Could you check a few things on this model? Use its own coordinates, in mm. A direction names the side the tool comes from. Round coordinates to 2 decimals unless told otherwise and drop trailing zeros. Write each loop counter-clockwise with the first axis right and the second up, starting at its lowest first coordinate (ties: lowest second). Pieces come first, ordered by that corner, then holes.
```python
from build123d import *

# Parameters (mm, degrees)
BOSS_EXTRUDE5_DEPTH = 10
BOSS_EXTRUDE6_DEPTH = 14.5
BOSS_EXTRUDE7_REACH = 63.425
SKETCH28_W          = 11
SKETCH28_H          = 29
SKETCH37_W          = 23.2
SKETCH37_H          = 14.666666667
CUT_EXTRUDE10_DEPTH = 6
SKETCH38_W          = 23.2
SKETCH38_H          = 5
CUT_EXTRUDE11_DEPTH = 6
SKETCH39_R          = 1.05
CUT_EXTRUDE12_DEPTH = 81.736980805
SKETCH40_R          = 2
CUT_EXTRUDE13_DEPTH = 1.4
SKETCH41_R          = 2
CUT_EXTRUDE14_DEPTH = 1.4
SKETCH42_W          = 17
SKETCH42_H          = 40
CUT_EXTRUDE15_DEPTH = 77.175521458
FILLET2_R           = 2
CUT_EXTRUDE16_DEPTH = 80.232001549
BOSS_EXTRUDE8_DEPTH = 10
FILLET3_R           = 10
FILLET4_R           = 5.45


with BuildPart() as part:
    # Sketch25 → Boss-Extrude5 (new, symmetric)
    with BuildSketch(Plane.XY):
        with BuildLine():
            Line((0, 15.875), (6.35, 15.875))
            ThreePointArc((6.35, 15.875), (9.840958299, 0), (6.35, -15.875))
            Line((6.35, -15.875), (0, -15.875))
            ThreePointArc((0, -15.875), (4.187196601, 0), (0, 15.875))
        make_face()
    extrude(amount=BOSS_EXTRUDE5_DEPTH, both=True)


with BuildPart() as body_2:
    # Sketch27 → Boss-Extrude6 (new, symmetric)
    with BuildSketch(Plane.XY):
        Polygon((0, -30.541666667), (11, -30.541666667), (11, -74.541666667), (0, -74.541666667), (0, -69.541666667), (6, -69.541666667), (6, -35.541666667), (0, -35.541666667), align=None)
    extrude(amount=BOSS_EXTRUDE6_DEPTH, both=True)

    # Sketch28 → Boss-Extrude7 (add, up to next)
    with BuildSketch(Plane.XZ.offset(15.875), mode=Mode.PRIVATE) as boss_extrude7_sk1:
        with Locations((5.5, 0)):
            Rectangle(SKETCH28_W, SKETCH28_H)
    boss_extrude7_tool1 = extrude(boss_extrude7_sk1.sketch, amount=BOSS_EXTRUDE7_REACH, mode=Mode.PRIVATE) - body_2.part

    add(part.part)  # Boss-Extrude7 merges part
    add(boss_extrude7_tool1.solids().sort_by_distance((5.5, -15.875, 0))[0])

    # Sketch37 → Cut-Extrude10 (cut)
    with BuildSketch(Plane.ZY):
        with Locations((0, -28.208333334)):
            Rectangle(SKETCH37_W, SKETCH37_H)
    extrude(amount=-CUT_EXTRUDE10_DEPTH, mode=Mode.SUBTRACT)

    # Sketch38 → Cut-Extrude11 (cut)
    with BuildSketch(Plane.ZY):
        with Locations((0, -72.041666667)):
            Rectangle(SKETCH38_W, SKETCH38_H)
    extrude(amount=-CUT_EXTRUDE11_DEPTH, mode=Mode.SUBTRACT)

    # Sketch39 → Cut-Extrude12 (cut, through all)
    with BuildSketch(Plane(origin=(0, 0, -14.5), x_dir=(-1, 0, 0), z_dir=(0, 0, -1))):
        with Locations((-2.5, -33.041666667)):
            Circle(SKETCH39_R)
        with Locations((-2.5, -72.041666667)):
            Circle(SKETCH39_R)
    extrude(amount=-CUT_EXTRUDE12_DEPTH, mode=Mode.SUBTRACT)

    # Sketch40 → Cut-Extrude13 (cut)
    with BuildSketch(Plane(origin=(0, 0, -14.5), x_dir=(-1, 0, 0), z_dir=(0, 0, -1))):
        with Locations((-2.5, -33.041666667)):
            Circle(SKETCH40_R)
        with Locations((-2.5, -72.041666667)):
            Circle(SKETCH40_R)
    extrude(amount=-CUT_EXTRUDE13_DEPTH, mode=Mode.SUBTRACT)

    # Sketch41 → Cut-Extrude14 (cut)
    with BuildSketch(Plane.XY.offset(14.5)):
        with Locations(Location((2.5, -33.041666667, 0), (0, 0, 180))):
            Circle(SKETCH41_R)
        with Locations(Location((2.5, -72.041666667, 0), (0, 0, 180))):
            Circle(SKETCH41_R)
    extrude(amount=-CUT_EXTRUDE14_DEPTH, mode=Mode.SUBTRACT)

    # Sketch42 → Cut-Extrude15 (cut, through all)
    with BuildSketch(Plane.ZY.offset(-6)):
        with Locations((0, -49.541666667)):
            Rectangle(SKETCH42_W, SKETCH42_H)
    extrude(amount=-CUT_EXTRUDE15_DEPTH, mode=Mode.SUBTRACT)

    # Fillet2
    fillet2_edges = [body_2.edges().sort_by_distance(p)[0] for p in [
        (8.5, -69.541666667, -8.5),
        (8.5, -29.541666667, -8.5),
        (8.5, -29.541666667, 8.5),
        (8.5, -69.541666667, 8.5),
        (0, -35.541666667, 13.05),
        (0, -69.541666667, 13.05),
        (0, -74.541666667, 13.05),
        (11, -74.541666667, 0),
        (0, -35.541666667, -13.05),
        (0, -74.541666667, -13.05),
        (0, -69.541666667, -13.05),
    ]]
    fillet(fillet2_edges, radius=FILLET2_R)

    # Sketch44 → Cut-Extrude16 (cut, through all)
    with BuildSketch(Plane.XY.offset(10)):
        with BuildLine():
            Line((6.35, -15.875), (0, -15.875))
            ThreePointArc((0, -15.875), (4.187196601, 0), (0, 15.875))
            Line((0, 15.875), (6.35, 15.875))
            ThreePointArc((6.35, 15.875), (9.840958299, 0), (6.35, -15.875))
        make_face()
    extrude(amount=-CUT_EXTRUDE16_DEPTH, mode=Mode.SUBTRACT)

    # Sketch43 → Boss-Extrude8 (add, symmetric)
    with BuildSketch(Plane.XY):
        with BuildLine():
            Line((-3.25, 15.875), (3.1, 15.875))
            ThreePointArc((3.1, 15.875), (6.232422098, 0), (3.1, -15.875))
            Line((3.1, -15.875), (-3.25, -15.875))
            ThreePointArc((-3.25, -15.875), (0.439252949, 0), (-3.25, 15.875))
        make_face()
    extrude(amount=BOSS_EXTRUDE8_DEPTH, both=True)

    # Fillet3
    # the kernel refuses this fillet: 10 mm, written as the material it takes off along each edge
    with BuildSketch(Plane(origin=(11, -15.875, 39.5), x_dir=(-1, 0, 0), z_dir=(0, 0, -1))) as fillet3_piece_1_section:
        with BuildLine():
            CenterArc((FILLET3_R, -FILLET3_R), FILLET3_R, 90, 90)
            Line((0, -FILLET3_R), (0, 0))
            Line((0, 0), (FILLET3_R, 0))
        make_face()
    fillet3_piece_1 = extrude(amount=79, mode=Mode.PRIVATE)
    fillet3_piece_1 = split(fillet3_piece_1, bisect_by=Plane(origin=(2.190951885, -15.815672455, 10), z_dir=(0, 0, 1)), keep=Keep.TOP, mode=Mode.PRIVATE)
    fillet3_piece_1 = fillet3_piece_1 & Plane(origin=(-35.560747051, 0, 24.75), x_dir=(0.925049424055658, 0.3798467625955178, 0), z_dir=(0, 0, 1)) * Cylinder(41.793169149, 198, mode=Mode.PRIVATE)
    add(fillet3_piece_1, mode=Mode.SUBTRACT)
    with BuildSketch(Plane(origin=(11, -15.875, 39.5), x_dir=(-1, 0, 0), z_dir=(0, 0, -1))) as fillet3_piece_2_section:
        with BuildLine():
            CenterArc((FILLET3_R, -FILLET3_R), FILLET3_R, 90, 90)
            Line((0, -FILLET3_R), (0, 0))
            Line((0, 0), (FILLET3_R, 0))
        make_face()
    fillet3_piece_2 = extrude(amount=79, mode=Mode.PRIVATE)
    fillet3_piece_2 = split(fillet3_piece_2, bisect_by=Plane(origin=(8.886802667, -18.192463431, 10), z_dir=(0, 0, 1)), keep=Keep.TOP, mode=Mode.PRIVATE)
    fillet3_piece_2 = fillet3_piece_2 - Plane(origin=(-35.560747051, 0, 24.75), x_dir=(0.925049424055658, 0.3798467625955178, 0), z_dir=(0, 0, 1)) * Cylinder(41.793169149, 198, mode=Mode.PRIVATE)
    add(fillet3_piece_2, mode=Mode.SUBTRACT)
    with BuildSketch(Plane(origin=(11, -15.875, 39.5), x_dir=(-1, 0, 0), z_dir=(0, 0, -1))) as fillet3_piece_3_section:
        with BuildLine():
            CenterArc((FILLET3_R, -FILLET3_R), FILLET3_R, 90, 90)
            Line((0, -FILLET3_R), (0, 0))
            Line((0, 0), (FILLET3_R, 0))
        make_face()
    fillet3_piece_3 = extrude(amount=79, mode=Mode.PRIVATE)
    fillet3_piece_3 = split(fillet3_piece_3, bisect_by=Plane(origin=(8.886802667, -18.192463431, 10), z_dir=(0, 0, -1)), keep=Keep.TOP, mode=Mode.PRIVATE)
    fillet3_piece_3 = fillet3_piece_3 - Plane(origin=(-35.560747051, 0, 0), x_dir=(0.925049424055658, 0.3798467625955178, 0), z_dir=(0, 0, 1)) * Cylinder(41.793169149, 198, mode=Mode.PRIVATE)
    fillet3_piece_3 = split(fillet3_piece_3, bisect_by=Plane(origin=(8.886802667, -18.192463431, -10), z_dir=(0, 0, 1)), keep=Keep.TOP, mode=Mode.PRIVATE)
    add(fillet3_piece_3, mode=Mode.SUBTRACT)
    with BuildSketch(Plane(origin=(11, -15.875, 39.5), x_dir=(-1, 0, 0), z_dir=(0, 0, -1))) as fillet3_piece_4_section:
        with BuildLine():
            CenterArc((FILLET3_R, -FILLET3_R), FILLET3_R, 90, 90)
            Line((0, -FILLET3_R), (0, 0))
            Line((0, 0), (FILLET3_R, 0))
        make_face()
    fillet3_piece_4 = extrude(amount=79, mode=Mode.PRIVATE)
    fillet3_piece_4 = fillet3_piece_4 & Plane(origin=(-35.560747051, 0, -24.75), x_dir=(0.925049424055658, 0.3798467625955178, 0), z_dir=(0, 0, 1)) * Cylinder(41.793169149, 198, mode=Mode.PRIVATE)
    fillet3_piece_4 = split(fillet3_piece_4, bisect_by=Plane(origin=(2.190951885, -15.815672455, -10), z_dir=(0, 0, -1)), keep=Keep.TOP, mode=Mode.PRIVATE)
    add(fillet3_piece_4, mode=Mode.SUBTRACT)
    with BuildSketch(Plane(origin=(11, -15.875, 39.5), x_dir=(-1, 0, 0), z_dir=(0, 0, -1))) as fillet3_piece_5_section:
        with BuildLine():
            CenterArc((FILLET3_R, -FILLET3_R), FILLET3_R, 90, 90)
            Line((0, -FILLET3_R), (0, 0))
            Line((0, 0), (FILLET3_R, 0))
        make_face()
    fillet3_piece_5 = extrude(amount=79, mode=Mode.PRIVATE)
    fillet3_piece_5 = fillet3_piece_5 - Plane(origin=(-35.560747051, 0, -24.75), x_dir=(0.925049424055658, 0.3798467625955178, 0), z_dir=(0, 0, 1)) * Cylinder(41.793169149, 198, mode=Mode.PRIVATE)
    fillet3_piece_5 = split(fillet3_piece_5, bisect_by=Plane(origin=(8.886802667, -18.192463431, -10), z_dir=(0, 0, -1)), keep=Keep.TOP, mode=Mode.PRIVATE)
    add(fillet3_piece_5, mode=Mode.SUBTRACT)

    # Fillet4
    # the kernel refuses this fillet: 5.45 mm, written as the material it adds along each edge
    with BuildSketch(Plane(origin=(0, -15.875, 10), x_dir=(-1, 0, 0), z_dir=(0, 0, -1))) as fillet4_piece_1:
        with BuildLine():
            CenterArc((5.45, -4.986231042), FILLET4_R, 113.807792078, 66.192207922)
            Line((0, -4.986231042), (0, 0))
            Line((0, 0), (3.25, 0))
        make_face()
    extrude(amount=20)
    with BuildSketch(Plane(origin=(3.015126937, -16.080140969, -10), x_dir=(0.33239794280209367, 0.9431392302417156, 0), z_dir=(0, 0, 1))) as fillet4_piece_2:
        with BuildLine():
            CenterArc((4.992113304, -5.441426809), FILLET4_R, 93.214160673, 71.449916977)
            ThreePointArc((-0.263821953, -4.000023125), (0.07058047, -2.013366907), (0, 0))
            ThreePointArc((0, 0), (2.343270621, -0.065743272), (4.686541241, 0))
        make_face()
    extrude(amount=20)


solid = body_2.part
```
Q1. If I drill on L1, parallel to Z at x = 8, y = -39.5; L2, parallel to Y at x = 2.5, z = 12.3; L3, parallel to Z at x = 5.5, y = -34, over which ranges is the centre line in solid material (lowest first)?
Q2. I'm going to push flat-ended pins straight in: pin 1 Ø2 at (x, y) = (2.5, -34) entering from -Z; pin 2 Ø1.5 at (x, z) = (4, -12.5) entering from +Y; pin 3 Ø1.3 at (x, y) = (2.5, -33.04) entering from -Z; pin 4 Ø5 at (y, z) = (-12.5, 2.5) entering from -X. Where does each tip first touch, or does it pass through?
Q3. On a 3-axis mill with a long thin cutter (end or side, diameter ignored), from which of +Z, -Z, +X, -X, +Y, -Y can I reach the whole of each face in a straight line? I mean faces 4 (the cylindrical face through (2.76, -31.06, -13.81)), 5 (the flat face through (8, -50, -8.5)), 6 (the flat face through (3, -28, -11.6)), 7 (the cylindrical face through (0.57, -70.143, 13.03)), 8 (the flat face through (1.6, -71.2, 13.1)). Say none if no direction works.
Q4. Imagine slicing it at B-B, the plane z = 1. Write out the boundary of the cut face in (x, y) (3 decimals), then the cut area to 3 significant figures.
Q5. We'd pull the mould along Z, two halves only. Please class faces 1 (the flat face through (4, -69.542, 13)), 2 (the flat face through (7, -45, 14.5)), 3 (the cylindrical face through (8.535, -30.143, 7.93)): pulls with the +Z half, pulls with the -Z half, needs draft (parallel to the pull), parting line crosses it, or undercut.
Q6. Imagine slicing it at A-A, the plane y = -51.5. Write out the boundary of the cut face in (x, z).
Q7. Imagine slicing it at D-D, the plane y = -14. Write out the boundary of the cut face in (x, z).
Q8. Imagine slicing it at C-C, the plane y = 2. Write out the boundary of the cut face in (x, z), then the cut area to 3 significant figures.
Results found:
1. L1: z = -14.5 to -8.5, 8.5 to 14.5
1. L2: y = -74.54 to -73.09, -70.99 to -69.54, -35.54 to -34.09, -31.99 to -15.99
1. L3: z = -14.5 to -11.6, 11.6 to 14.5
2. pin 1: stops at z = -13.1
2. pin 2: stops at y = -16.13
2. pin 3: passes through
2. pin 4: stops at x = -2.83
3. face 4: -Z
3. face 5: +X, -X
3. face 6: -X, -Y
3. face 7: +Z, -Z, -X
3. face 8: +Z
4. outline: (-3.25, -15.875) arc R5.45 cw to (0, -20.861) - (0, -20.875) - (6, -20.875) - (6, -29.542) - (11, -29.542) - (11, -25.875) arc R10 ccw to (6.7, -17.659) arc R5.45 cw to (4.573, -11.66) arc R41.793 ccw to (3.1, 15.875) - (-3.25, 15.875) arc R36 cw to start; (6, -74.542) - (9, -74.542) arc R2 ccw to (11, -72.542) - (11, -69.542) - (6, -69.542) - close
4. area: 299 mm2
5. face 1: needs draft
5. face 2: pulls with the +Z half
5. face 3: undercut
6. outline: (6, -14.5) - (11, -14.5) - (11, -8.5) - (6, -8.5) - close; (6, 8.5) - (11, 8.5) - (11, 14.5) - (6, 14.5) - close
7. outline: (-2.39, -10) - (4.42, -10) - (4.42, 10) - (-2.39, 10) - close
8. outline: (0.38, -10) - (6.18, -10) - (6.18, 10) - (0.38, 10) - close
8. area: 116 mm2
